from build123d import *

# Parameters (mm, degrees)
ESBO_O1_W                  = 63.3
ESBO_O1_H                  = 45
ESBO_O1_R                  = 11.5
ESBO_O1_R_2                = 1.75
ESBO_O1_R_3                = 1.65
RESSALTO_EXTRUS_O1_DEPTH   = 25
CORTE_EXTRUS_O1_DEPTH      = 54.262932702
CORTE_EXTRUS_O1_DEPTH_BACK = 54.262932702
ESBO_O2_W                  = 13.3
ESBO_O2_H                  = 21


with BuildPart() as part:
    # Esboço1 → Ressalto-extrusão1 (new body)
    with BuildSketch(Plane.XY):
        with Locations((-9.65, 0)):
            Rectangle(ESBO_O1_W, ESBO_O1_H)
        Circle(ESBO_O1_R, mode=Mode.SUBTRACT)
        with Locations((-15.5, 15.5)):
            Circle(ESBO_O1_R_2, mode=Mode.SUBTRACT)
        with Locations((15.5, 15.5)):
            Circle(ESBO_O1_R_2, mode=Mode.SUBTRACT)
        with Locations((15.5, -15.5)):
            Circle(ESBO_O1_R_2, mode=Mode.SUBTRACT)
        with Locations((-15.5, -15.5)):
            Circle(ESBO_O1_R_2, mode=Mode.SUBTRACT)
        with Locations((-31.3, -15.5)):
            Circle(ESBO_O1_R_3, mode=Mode.SUBTRACT)
        with Locations((-31.3, 15.5)):
            Circle(ESBO_O1_R_3, mode=Mode.SUBTRACT)
    extrude(amount=RESSALTO_EXTRUS_O1_DEPTH)

    # Esboço2 → Corte-extrusão1 (cut, two sides: drawn at the far end of the back side and taken through both)
    with BuildSketch(Plane(origin=(0, 0, 0), x_dir=(1, 0, 0), z_dir=(0, 1, 0)).offset(-CORTE_EXTRUS_O1_DEPTH_BACK)):
        with Locations((-34.65, -14.5)):
            Rectangle(ESBO_O2_W, ESBO_O2_H)
        Polygon((-23, -25), (22, -25), (22, -4), align=None)
        Polygon((-23, -25), (22, -4), (-23, -4), (-28, -4), (-28, -25), align=None)
    extrude(amount=CORTE_EXTRUS_O1_DEPTH + CORTE_EXTRUS_O1_DEPTH_BACK, mode=Mode.SUBTRACT)


solid = part.part
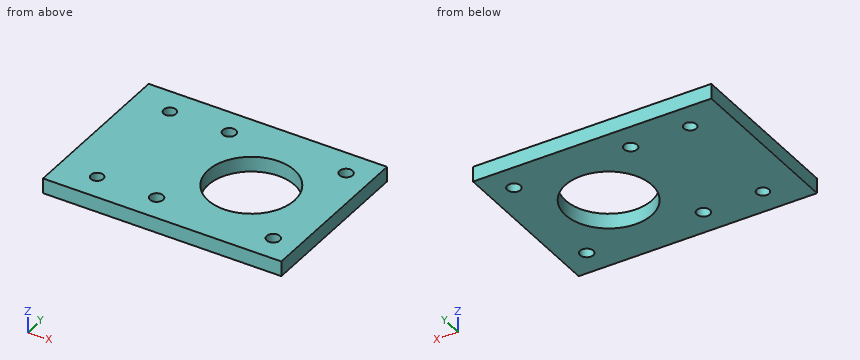
The listing builds one solid part. Answer for the finished solid, in the listing's coordinates (mm). Give positions to 0.01 mm unless a question says otherwise; leave off trailing zeros. Order: outer loops, then holes, each group sorted by start corner. A loop starts at its lowest first (then second) coordinate and runs counter-clockwise, first axis right, second up. Notation, with made-up numbers: (46.25, 34.25) -> (65.25, 34.25) arc R16 cw to (65.25, 51.25) -> close; hole circle Ø5 at (84, 70.5). An arc over 180 degrees is marked (long way). Put each result on its own line as item: value.
Item 1: Straight lines are drawn through the part: line 1 (X direction, y = -15.5, z = 2.6); line 2 (Y direction, x = -15.5, z = 0.85); line 3 (Y direction, x = 0, z = 1.65). For each, find the intervals that lie inside material, in ascending order.
Established:
line 1: x = -41.3 to -32.95, -29.65 to -17.25, -13.75 to 13.75, 17.25 to 22
line 2: y = -22.5 to -17.25, -13.75 to 13.75, 17.25 to 22.5
line 3: y = -22.5 to -11.5, 11.5 to 22.5
Item 2: A cutting plane is placed at B-B on z = 3.2. Give the vertices of the cut face in (x, y).
Established:
outline: (-41.3, -22.5) -> (22, -22.5) -> (22, 22.5) -> (-41.3, 22.5) -> close; hole circle Ø3.3 at (-31.3, -15.5); hole circle Ø3.3 at (-31.3, 15.5); hole circle Ø3.5 at (-15.5, -15.5); hole circle Ø3.5 at (-15.5, 15.5); hole circle Ø23 at (0, 0); hole circle Ø3.5 at (15.5, -15.5); hole circle Ø3.5 at (15.5, 15.5)
Item 3: Given P1, Ø3, axis at x = -15.5, y = 15.5, coming from the -Z side (3 decimals), flat-ended and moving along its own axis, determine where the tip first touches the part or whether it passes through.
Established:
P1: passes through
Item 4: A cutting plane is placed at D-D on y = 15.5. Give the vertices of the cut face in (x, z).
Established:
outline: (-41.3, 0) -> (-32.95, 0) -> (-32.95, 4) -> (-41.3, 4) -> close; (-29.65, 0) -> (-17.25, 0) -> (-17.25, 4) -> (-29.65, 4) -> close; (-13.75, 0) -> (13.75, 0) -> (13.75, 4) -> (-13.75, 4) -> close; (17.25, 0) -> (22, 0) -> (22, 4) -> (17.25, 4) -> close
Item 5: A cutting plane is placed at A-A on x = -15.5. Give the vertices of the cut face in (y, z), plus the area to 3 significant figures.
Established:
outline: (-22.5, 0) -> (-17.25, 0) -> (-17.25, 4) -> (-22.5, 4) -> close; (-13.75, 0) -> (13.75, 0) -> (13.75, 4) -> (-13.75, 4) -> close; (17.25, 0) -> (22.5, 0) -> (22.5, 4) -> (17.25, 4) -> close
area: 152 mm^2
Item 6: A cutting plane is placed at C-C on y = 0. Give the vertices of the cut face in (x, z).
Established:
outline: (-41.3, 0) -> (-11.5, 0) -> (-11.5, 4) -> (-41.3, 4) -> close; (11.5, 0) -> (22, 0) -> (22, 4) -> (11.5, 4) -> close
